Model file for the job. Use its own axes, mm. Face numbers are marked on the shaded views. Coordinates: 2 decimals unless noted, no trailing zeros. Loops run counter-clockwise (first coordinate to the right, second up) from the corner with the lowest first, then second, coordinate; pieces in that order, holes last.
from build123d import *

# Parameters (mm, degrees)
SKETCH1_W           = 140.676923077
SKETCH1_H           = 1.27
BOSS_EXTRUDE1_DEPTH = 12.7
SKETCH1_3_W         = 140.676923077
SKETCH1_3_H         = 60.96
BOSS_EXTRUDE2_DEPTH = 1.27
SKETCH2_R           = 3.175
CUT_EXTRUDE1_DEPTH  = 508
SKETCH1_5_W         = 140.676923077
SKETCH1_5_H         = 1.27
BOSS_EXTRUDE3_DEPTH = 12.7
SKETCH3_R           = 3.175
CUT_EXTRUDE2_DEPTH  = 12.7
FILLET1_R           = 6.35
FILLET2_R           = 0.635
SKETCH3_2_R         = 3.175
CUT_EXTRUDE3_DEPTH  = 155.866189617


with BuildPart() as part:
    # Sketch1 → Boss-Extrude1 (new body)
    with BuildSketch(Plane(origin=(0, 0, 0), x_dir=(1, 0, 0), z_dir=(0, 1, 0))):
        with Locations((70.338461538, 0.635)):
            Rectangle(SKETCH1_W, SKETCH1_H)
    extrude(amount=BOSS_EXTRUDE1_DEPTH)

    # Sketch1<3> → Boss-Extrude2 (add)
    with BuildSketch(Plane(origin=(0, 0, 0), x_dir=(1, 0, 0), z_dir=(0, 1, 0))):
        with Locations((70.338461538, 31.75)):
            Rectangle(SKETCH1_3_W, SKETCH1_3_H)
    extrude(amount=BOSS_EXTRUDE2_DEPTH)

    # Sketch2 → Cut-Extrude1 (cut)
    with BuildSketch(Plane.XY):
        with Locations((6.37364392, 6.35)):
            Circle(SKETCH2_R)
        with Locations((146.05, 6.35)):
            Circle(SKETCH2_R)
    extrude(amount=-CUT_EXTRUDE1_DEPTH, mode=Mode.SUBTRACT)

    # Sketch1<5> → Boss-Extrude3 (add)
    with BuildSketch(Plane(origin=(0, 0, 0), x_dir=(1, 0, 0), z_dir=(0, 1, 0))):
        with Locations((70.338461538, 62.865)):
            Rectangle(SKETCH1_5_W, SKETCH1_5_H)
    extrude(amount=BOSS_EXTRUDE3_DEPTH)

    # Sketch3 → Cut-Extrude2 (cut)
    with BuildSketch(Plane(origin=(0, 0, -63.5), x_dir=(-1, 0, 0), z_dir=(0, 0, -1))):
        with Locations((-6.35, 6.35)):
            Circle(SKETCH3_R)
        with Locations((-146.05, 6.35)):
            Circle(SKETCH3_R)
        with Locations((-134.326923077, 6.35)):
            Circle(SKETCH3_R)
    extrude(amount=-CUT_EXTRUDE2_DEPTH, mode=Mode.SUBTRACT)

    # Fillet1
    fillet1_edges = [part.edges().sort_by_distance(p)[0] for p in [
        (0, 12.7, -0.635),
        (140.676923077, 12.7, -0.635),
        (0, 12.7, -62.865),
        (140.676923077, 12.7, -62.865),
    ]]
    fillet(fillet1_edges, radius=FILLET1_R)

    # Fillet2
    fillet2_edges = [part.edges().sort_by_distance(p)[0] for p in [
        (70.338461538, 1.27, -62.23),
        (70.338461538, 1.27, -1.27),
    ]]
    fillet(fillet2_edges, radius=FILLET2_R)

    # Sketch3<2> → Cut-Extrude3 (cut, through all)
    with BuildSketch(Plane(origin=(0, 0, -63.5), x_dir=(-1, 0, 0), z_dir=(0, 0, -1))):
        with Locations((-6.35, 6.35)):
            Circle(SKETCH3_2_R)
        with Locations((-146.05, 6.35)):
            Circle(SKETCH3_2_R)
        with Locations((-134.326923077, 6.35)):
            Circle(SKETCH3_2_R)
    extrude(amount=-CUT_EXTRUDE3_DEPTH, mode=Mode.SUBTRACT)


solid = part.part
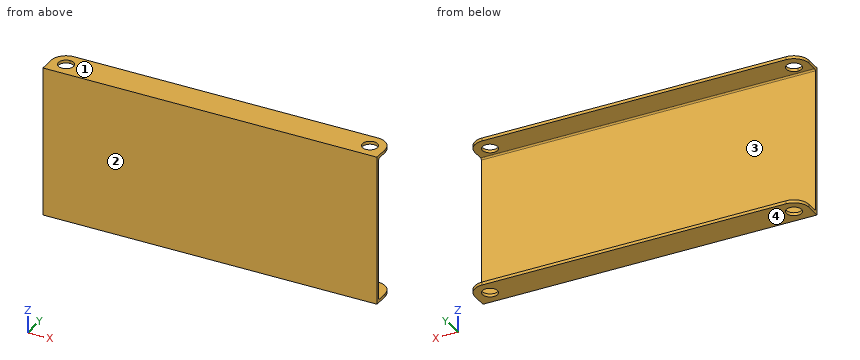
Q1. Slice it at A-A (y = 4.5). List the corners of the cut face in (x, z).
Answers:
outline: (0, -63.5) - (3.77, -63.5) - (3.77, -62.23) - (0, -62.23) - close; (0, -1.27) - (3.77, -1.27) - (3.77, 0) - (0, 0) - close; (8.93, -63.5) - (131.75, -63.5) - (131.75, -62.23) - (8.93, -62.23) - close; (8.95, -1.27) - (131.75, -1.27) - (131.75, 0) - (8.95, 0) - close; (136.91, -63.5) - (140.68, -63.5) - (140.68, -62.23) - (136.91, -62.23) - close; (136.91, -1.27) - (140.68, -1.27) - (140.68, 0) - (136.91, 0) - close
Q2. Slice it at C-C (z = -32.5). List the corners of the cut face in (x, y), and give its area (3 significant figures).
Answers:
outline: (0, 0) - (140.68, 0) - (140.68, 1.27) - (0, 1.27) - close
area: 179 mm2
Q3. Drill centre lines: line 1 (Z direction, x = 73.5, y = 5.5); line 2 (Y direction, x = 134, z = -20.5). Where is each one in solid material? Low to high.
Answers:
line 1: z = -63.5 to -62.23, -1.27 to 0
line 2: y = 0 to 1.27
Q4. Slice it at B-B (x = 96). List the corners of the cut face in (y, z) (3 decimals), and give its area (3 significant figures).
Answers:
outline: (0, -63.5) - (12.7, -63.5) - (12.7, -62.23) - (1.905, -62.23) arc R0.635 cw to (1.27, -61.595) - (1.27, -1.905) arc R0.635 cw to (1.905, -1.27) - (12.7, -1.27) - (12.7, 0) - (0, 0) - close
area: 110 mm2
Q5. Mould opens along Z. For the marked faces 1, 2, 3 and 4 say: +Z half, -Z half, draft (parallel to the pull), parting line (faces both ways), or undercut.
Answers:
face 1: +Z half
face 2: draft
face 3: undercut
face 4: -Z half
